Read the model definition and answer for the solid it produces. Units are mm, in the model's axes. Face numbers are marked on the shaded views. A direction names the side the tool comes from. Round coordinates to 2 decimals unless told otherwise and drop trailing zeros. Loops run counter-clockwise (first coordinate to the right, second up) from the corner with the lowest first, then second, coordinate; pieces in that order, holes last. Notation, with made-up numbers: M 31.5,81.25 L 74.5,81.25 A22 ccw 74.5,104.25 Z; hole C 21.5,-32.75 d10. An arc over 180 degrees is marked long. Write each question's results on one line, items separated by ' | '.
```python
from build123d import *

# Parameters (mm, degrees)
F0_W     = 76.2
F0_H     = 76.2
F1_DEPTH = 19.05
F3_DEPTH = 76.2
F4_W     = 76.2
F4_H     = 76.2
F4_R     = 21.6703506802
F5_DEPTH = 19.05
F7_DEPTH = 114.301


with BuildPart() as f1:
    # F0 (on Front) → F1 (new body)
    with BuildSketch(Plane.XZ):
        with Locations((-23.25902578, 1.1713085696)):
            Rectangle(F0_W, F0_H)
    extrude(amount=-F1_DEPTH)

    # F2 (on face) → F3 (join)
    with BuildSketch(Plane.XZ):
        with BuildLine():
            Line((-38.5822776966, 16.4945604863), (-7.9357738633, -14.1519433471))
            ThreePointArc((-7.9357738633, -14.1519433471), (-3.2382323242, -7.1215756093), (-1.5886750997, 1.1713085696))
            ThreePointArc((-1.5886750997, 1.1713085696), (-14.9661416011, 21.1921020254), (-38.5822776966, 16.4945604863))
        make_face()
        with BuildLine():
            ThreePointArc((-38.5822776966, 16.4945604863), (-38.5822776966, -14.1519433471), (-7.9357738633, -14.1519433471))
            Line((-7.9357738633, -14.1519433471), (-38.5822776966, 16.4945604863))
        make_face()
    extrude(amount=F3_DEPTH)

    # F4 (on face) → F5 (join)
    with BuildSketch(Plane.XZ.offset(76.2)):
        with Locations((-22.6412163979, 0.4432164133)):
            Rectangle(F4_W, F4_H)
        with Locations((-23.25902578, 1.1713085696)):
            Circle(F4_R)
    extrude(amount=F5_DEPTH)

    # F6 (on face) → F7 (cut, through all)
    with BuildSketch(Plane.XZ.offset(95.25)):
        with BuildLine():
            ThreePointArc((-3.5912163979, 0.4432164133), (-5.0413113036, 7.7333357998), (-9.1708322163, 13.9136005949))
            Line((-9.1708322163, 13.9136005949), (-22.6412163979, 0.4432164133))
            Line((-22.6412163979, 0.4432164133), (-9.1708322163, -13.0271677683))
            ThreePointArc((-9.1708322163, -13.0271677683), (-5.0413113036, -6.8469029733), (-3.5912163979, 0.4432164133))
        make_face()
        with BuildLine():
            Line((-22.6412163979, 0.4432164133), (-9.1708322163, 13.9136005949))
            ThreePointArc((-9.1708322163, 13.9136005949), (-22.6412163979, 19.4932164133), (-36.1116005795, 13.9136005949))
            Line((-36.1116005795, 13.9136005949), (-22.6412163979, 0.4432164133))
        make_face()
        with BuildLine():
            Line((-9.1708322163, -13.0271677683), (-22.6412163979, 0.4432164133))
            Line((-22.6412163979, 0.4432164133), (-36.1116005795, -13.0271677683))
            ThreePointArc((-36.1116005795, -13.0271677683), (-22.6412163979, -18.6067835867), (-9.1708322163, -13.0271677683))
        make_face()
        with BuildLine():
            Line((-36.1116005795, -13.0271677683), (-22.6412163979, 0.4432164133))
            Line((-22.6412163979, 0.4432164133), (-36.1116005795, 13.9136005949))
            ThreePointArc((-36.1116005795, 13.9136005949), (-41.6912163979, 0.4432164133), (-36.1116005795, -13.0271677683))
        make_face()
    extrude(amount=-F7_DEPTH, mode=Mode.SUBTRACT)


solid = f1.part
```
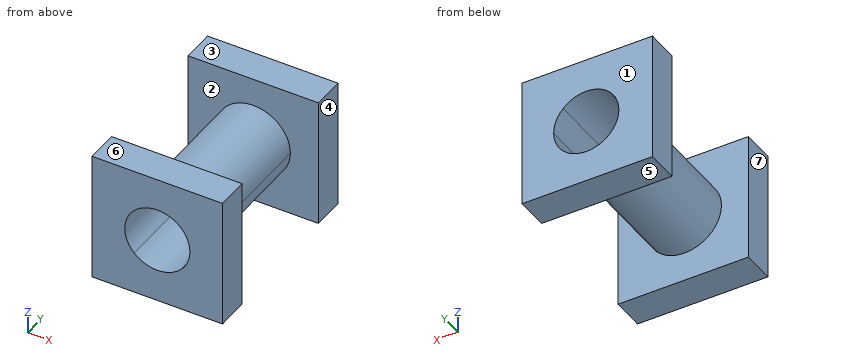
1. Determine the mould class of the marked faces 1, 2 and 3 for opening direction Y: released by +Y, released by -Y, zero draft, split by the parting line, or undercut.
Completed:
face 1: released by +Y | face 2: undercut | face 3: zero draft
2. Find section B-B, the plane y = -42. Give the vertices of the cut face in (x, z), then the cut area to 3 significant figures.
Completed:
outline: C -23.26,1.17 d43.34; hole C -22.64,0.44 d38.1 | area: 335 mm2
3. Find section D-D, the plane z = -11. Give the vertices of the cut face in (x, y), then the cut area to 3 significant figures.
Completed:
outline: M -61.36,0 L -41.19,0 L -41.19,-76.2 L -60.74,-76.2 L -60.74,-95.25 L -37.87,-95.25 L -37.87,19.05 L -61.36,19.05 Z; M -7.41,-95.25 L 15.46,-95.25 L 15.46,-76.2 L -5.33,-76.2 L -5.33,0 L 14.84,0 L 14.84,19.05 L -7.41,19.05 Z | area: 2,150 mm2
4. Find section C-C, the plane x = -54. Give the vertices of the cut face in (y, z).
Completed:
outline: M -95.25,-37.66 L -76.2,-37.66 L -76.2,38.54 L -95.25,38.54 Z; M 0,-36.93 L 19.05,-36.93 L 19.05,39.27 L 0,39.27 Z
5. Given P1, Ø15, axis at x = -12, y = -83, coming from the +Z side; P2, Ø9.5, axis at y = -89.5, z = 15.5, coming from the -X side; P3, Ø6, axis at y = -48.5, z = 19.5, coming from the -X side, each flat-ended and moving along its own axis, determine where each tip first touches the part or whether it passes through.
Completed:
P1: stops at z = 38.54 | P2: stops at x = -60.74 | P3: stops at x = -38.58
6. Find the intervals of material crossed by L1, parallel to Y at x = -13.5, z = 34; L2, parallel to X at y = -64, z = -9; L3, parallel to X at y = -1, z = -1.5, in increasing order.
Completed:
L1: y = -95.25 to -76.2, 0 to 19.05 | L2: x = -42.39 to -39.19, -6.1 to -4.12 | L3: x = -44.76 to -41.59, -3.69 to -1.75
7. Which of the six approach directions +Z, -Z, +X, -X, +Y, -Y give full straight-line access (tool end or side, diameter ignored) to the marked faces 4, 5, 6 and 7?
Completed:
face 4: +Z, -Z, +X, +Y | face 5: -Z, +X, -X, +Y | face 6: +Z, +X, -X, -Y | face 7: +Z, -Z, -X, -Y
8. Find section A-A, the plane z = 29.5. Give the vertices of the cut face in (x, y), then the cut area to 3 significant figures.
Completed:
outline: M -61.36,0 L 14.84,0 L 14.84,19.05 L -61.36,19.05 Z; M -60.74,-95.25 L 15.46,-95.25 L 15.46,-76.2 L -60.74,-76.2 Z | area: 2,900 mm2
